from build123d import *

# Parameters (mm, degrees)
F0_R = 34.2479621902


with BuildPart() as f2:
    # F2: sweep along a path in F1
    with BuildLine(Plane.YZ) as f2_path:
        Line((0, 0), (0, 42.1044450237))
        ThreePointArc((0, 42.1044450237), (-5.6069266237, 65.3041458582), (-21.1900046775, 83.3826254221))
        Line((-21.1900046775, 83.3826254221), (-36.5290609103, 94.3857602241))
        ThreePointArc((-36.5290609103, 94.3857602241), (-42.763778711, 98.2100897423), (-49.4830708618, 101.0994348776))
        Line((-49.4830708618, 101.0994348776), (-160.7226986152, 139.7061028327))
        ThreePointArc((-160.7226986152, 139.7061028327), (-206.7855450766, 146.6494265049), (-252.25333688, 136.5165356896))
        Line((-252.25333688, 136.5165356896), (-368.6925900292, 86.7757238812))
        ThreePointArc((-368.6925900292, 86.7757238812), (-390.1894627935, 69.4242484731), (-399.4271314968, 43.3886053197))
        Line((-399.4271314968, 43.3886053197), (-405.4229263948, -47.9120732419))
        ThreePointArc((-405.4229263948, -47.9120732419), (-391.8386577153, -96.5654209485), (-350.8094442607, -126.0320841785))
        Line((-350.8094442607, -126.0320841785), (-225.1088500457, -162.8565612302))
    # F0 (on Top) → F2 (sweep)
    with BuildSketch(Plane.XY):
        Circle(F0_R)
    sweep(path=f2_path.line)


solid = f2.part
Can you work these out from the model? Positions are in its coordinate system, mm. A direction names the side the tool comes from. Give positions to 0.01 mm unless a question says otherwise; leave off trailing zeros. Loops run counter-clockwise (first coordinate to the right, second up) from the corner with the lowest first, then second, coordinate; pieces in that order, holes last. Notation, with made-up numbers: (67, 72.25) -> (83, 72.25) arc R27 ccw to (83, 110.25) -> close; hole circle Ø6 at (50, 2.5). An arc over 180 degrees is marked (long way). Return JSON: item names as keys, results as strings.
Q1. For pin 1 Ø1.5 at (x, y) = (1, -96.5) entering from +Z; pin 2 Ø2 at (x, z) = (-12.5, 70.5) entering from -Y, each with a flat end and sliding along its axis, tell me the tip position at first contact or that it passes through.
Checks:
{"pin 1": "stops at z = 153.91", "pin 2": "stops at y = -426.18"}
Q2. I need wall thicknesses on probe 1 along Z at (x, y) = (-26, -306); probe 2 along Z at (x, y) = (-30, -266); probe 3 along Y at (x, z) = (29, 6.5). Which ranges of each line are inside material? Lowest first, please.
Checks:
{"probe 1": "z = -162.39 to -115.93, 89.32 to 137.8", "probe 2": "z = -168.09 to -133.66, 112.68 to 148.61", "probe 3": "y = -420.11 to -383.59, -18.22 to 18.22"}
Q3. I want a section at A-A, the plane x = 15.5. List the corners of the cut face in (y, z) for me.
Checks:
{"outline": "(-435.9, -45.91) arc R106.74 ccw to (-359.4, -155.34) -> (-233.69, -192.16) -> (-216.52, -133.55) -> (-342.22, -96.72) arc R45.66 cw to (-374.95, -49.91) -> (-368.95, 41.39) arc R20.26 cw to (-356.7, 58.69) -> (-240.26, 108.43) arc R96.46 cw to (-170.74, 110.85) -> (-59.5, 72.25) arc R20.26 cw to (-54.33, 69.57) -> (-38.99, 58.57) arc R20.26 cw to (-30.54, 42.1) -> (-30.54, 0) -> (30.54, 0) -> (30.54, 42.1) arc R81.34 ccw to (-3.39, 108.2) -> (-18.73, 119.2) arc R81.34 ccw to (-39.47, 129.95) -> (-150.71, 168.56) arc R157.54 ccw to (-264.25, 164.6) -> (-380.69, 114.86) arc R81.34 ccw to (-429.9, 45.39) -> close"}
Q4. On a 3-axis mill with a long thin cutter (end or side, diameter ignored), from which of +Z, -Z, +X, -X, +Y, -Y can I reach the whole of each face in a straight line? I mean faces 1 (the face through (-4.458, 33.957, 21.347)), 2 (the face through (-7.424, -298.154, 80.552)). Say none if no direction works.
Checks:
{"face 1": "-Z", "face 2": "none"}
Q5. We'd pull the mould along Z, two halves only. Please class faces 3 (the face through (32.666, -22.971, 97.32)), 4 (the face through (0, 0, 0)), 5 (the face through (-4.46, -436.35, -0.68)): released by +Z, released by -Z, zero draft, split by the parting line, or undercut.
Checks:
{"face 3": "split by the parting line", "face 4": "released by -Z", "face 5": "undercut"}
